Geometry check sheet. Reference: the model listing, model coordinates, mm. Coordinates: 2 decimals unless noted, no trailing zeros. Write each loop counter-clockwise with the first axis right and the second up, starting at its lowest first coordinate (ties: lowest second). Pieces come first, ordered by that corner, then holes. Notation, with made-up numbers: (1, 66.25) -> (12, 66.25) arc R24 cw to (12, 100.25) -> close; hole circle Ø4 at (1.25, 71). An arc over 180 degrees is marked (long way). Use a Markdown table: item, result.
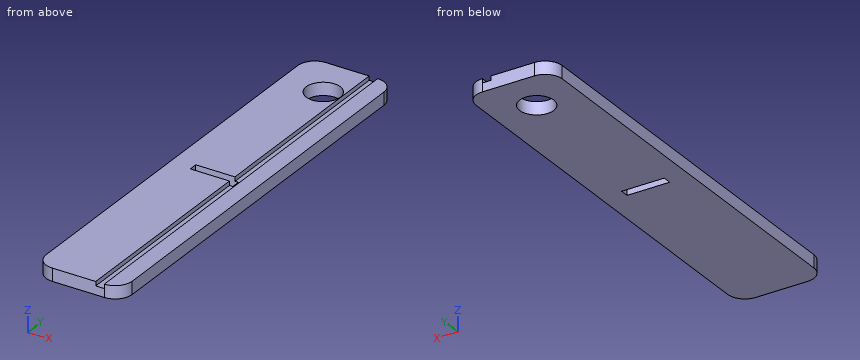
Autodesk Fusion 360 part; units mm, degrees
sketch "Sketch1" plane through (0, 0, 0) normal (0, 0, 1) x (1, 0, 0)
  line L0 (0, 0) -> (20.2, 0)
  line L1 (20.2, 0) -> (20.2, 100.2)
  line L2 (20.2, 100.2) -> (0, 100.2)
  line L3 (0, 100.2) -> (0, 0)
  circle A0 centre (10.1, 89.7864) radius 4
  line L4 (15, 51) -> (5, 51)
  line L5 (5, 51) -> (5, 49)
  line L6 (5, 49) -> (15, 49)
  line L7 (15, 49) -> (15, 51)
  line L8 (15, 51) -> (5, 49) construction
  line L9 (5, 51) -> (15, 49) construction
  line L10 (10.1, 100.2) -> (10.1, 0) construction
  point P0 (10, 50)
  dimension "d1" = 20.2
  dimension "d2" = 100.2
  dimension "d8" = 8
  dimension "d9" = 10
  dimension "d10" = 2
extrude "Extrude1" add sketch "Sketch1" along normal blind 3
fillet "Fillet1" radius 4 4 edges at (20.2, 0, 1.5) (20.2, 100.2, 1.5) (0, 100.2, 1.5) (0, 0, 1.5)
sketch "Sketch2" plane through (0, 0, 3) normal (0, 0, 1) x (-1, 0, 0)
  arc A0 (0, -4) -> (-4, 0) centre (-4, -4) ccw
  line L0 (-4, 0) -> (-16.2, 0)
  arc A1 (-16.2, 0) -> (-20.2, -4) centre (-16.2, -4) ccw
  line L1 (-20.2, -4) -> (-20.2, -96.2)
  arc A2 (-20.2, -96.2) -> (-16.2, -100.2) centre (-16.2, -96.2) ccw
  line L2 (-16.2, -100.2) -> (-4, -100.2)
  arc A3 (-4, -100.2) -> (0, -96.2) centre (-4, -96.2) ccw
  line L3 (0, -96.2) -> (0, -4)
  line L4 (-15, -51) -> (-15, -49)
  line L5 (-15, -49) -> (-5, -49)
  line L6 (-5, -49) -> (-5, -51)
  line L7 (-5, -51) -> (-15, -51)
  circle A4 centre (-10.1, -89.7864) radius 4
  line L8 (-16.2, 0) -> (-14.2, 0)
  line L9 (-14.2, 0) -> (-14.2, -100.2)
  line L10 (-14.2, -100.2) -> (-16.2, -100.2)
  line L11 (-16.2, -100.2) -> (-16.2, 0)
  dimension "d11" = 2
extrude "Extrude2" cut sketch "Sketch2" against normal blind 1 contours L0 L2 L4 L5 L7 L8 L9 L10 L11
Item 1: Section check A-A on x = 10.1. Record the boundary of the cut face in (y, z), then the cut area to 3 significant figures.
Answer block:
| item | result |
|---|---|
| outline | (0, 0) -> (49, 0) -> (49, 3) -> (0, 3) -> close; (51, 0) -> (85.79, 0) -> (85.79, 3) -> (51, 3) -> close; (93.79, 0) -> (100.2, 0) -> (100.2, 3) -> (93.79, 3) -> close |
| area | 271 mm^2 |
Item 2: Section check B-B on y = 66. Record the boundary of the cut face in (x, z), then the cut area to 3 significant figures.
Answer block:
| item | result |
|---|---|
| outline | (0, 0) -> (20.2, 0) -> (20.2, 3) -> (16.2, 3) -> (16.2, 2) -> (14.2, 2) -> (14.2, 3) -> (0, 3) -> close |
| area | 58.6 mm^2 |
Item 3: Thickness scan on L1, parallel to Y at x = 10.1, z = 2.15; L2, parallel to X at y = 58, z = 2.9; L3, parallel to Y at x = 6, z = 2.85. Record the ranges inside material, lowest first. Write a range as [from, to].
Answer block:
| item | result |
|---|---|
| L1 | y = [0, 49], [51, 85.79], [93.79, 100.2] |
| L2 | x = [0, 14.2], [16.2, 20.2] |
| L3 | y = [0, 49], [51, 100.2] |
Item 4: Section check C-C on z = 0.95. Record the boundary of the cut face in (x, y), then the cut area to 3 significant figures.
Answer block:
| item | result |
|---|---|
| outline | (0, 4) arc R4 ccw to (4, 0) -> (16.2, 0) arc R4 ccw to (20.2, 4) -> (20.2, 96.2) arc R4 ccw to (16.2, 100.2) -> (4, 100.2) arc R4 ccw to (0, 96.2) -> close; hole (5, 49) -> (15, 49) -> (15, 51) -> (5, 51) -> close; hole circle Ø8 at (10.1, 89.79) |
| area | 1,940 mm^2 |
